Source: three-view drawing plus pictorial views. Frame: mm from the lowest corner of the part. A direction names the side the tool comes from. Give positions to 0.01 mm unless a question says otherwise; leave off trailing zeros. Order: outer loops, then holes, each group sorted by start corner. A loop starts at its lowest first (then second) coordinate and runs counter-clockwise, first axis right, second up.
1) Material intervals for line 1 (Y direction, x = 6.5, z = 12); line 2 (X direction, y = 66, z = 13); line 3 (Z direction, x = 22, y = 33), sorted ascending.
2) First-contact query: P1, Ø12, axis at x = 33, z = 15.5, coming from the -Y side. Flat tip, straight axial feed; report the tip coordinate or a pass-through.
3) Section C-C, the plane y = 22.5. Return loops of the section in (x, z).
4) Section B-B, the plane x = 30. Return loops of the section in (y, z), plus the area to 3 significant figures.
5) Draft query along X for the marked faces 4, 5 and 6. Return one class per face: released by +X, released by -X, zero draft, split by the parting line, or undercut.
6) Section A-A, the plane z = 23. Return loops of the section in (x, y), plus the area to 3 significant figures.
7) Access query for the marked faces 1, 2 and 3. Directions: +Z, -Z, +X, -X, +Y, -Y. A direction counts if a zero-diameter tool reaches every point of the face in a straight line with its end or side. Return the directions, or none.
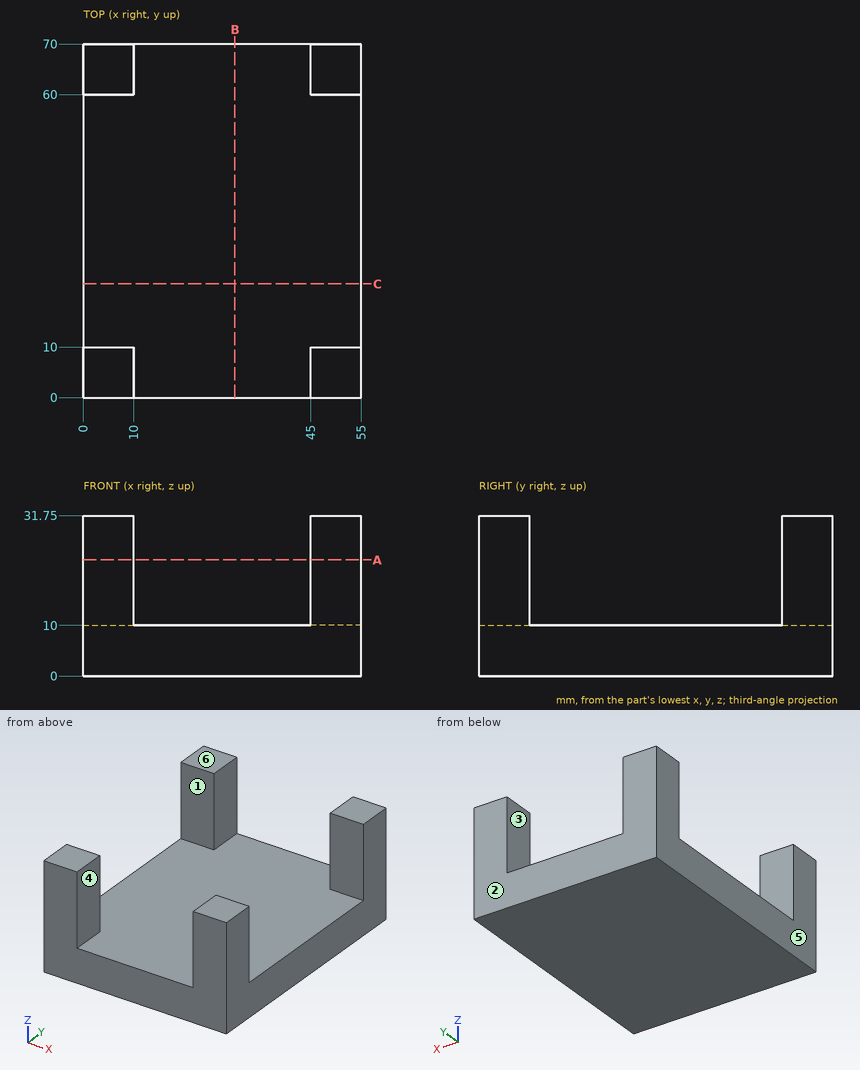
From the geometry:
1. line 1: y = 0 to 10, 60 to 70
1. line 2: x = 0 to 10, 45 to 55
1. line 3: z = 0 to 10
2. P1: stops at y = 0
3. outline: (0, 0) - (55, 0) - (55, 10) - (0, 10) - close
4. outline: (0, 0) - (70, 0) - (70, 10) - (0, 10) - close
4. area: 700 mm2
5. face 4: undercut
5. face 5: released by -X
5. face 6: zero draft
6. outline: (0, 0) - (10, 0) - (10, 10) - (0, 10) - close; (0, 60) - (10, 60) - (10, 70) - (0, 70) - close; (45, 0) - (55, 0) - (55, 10) - (45, 10) - close; (45, 60) - (55, 60) - (55, 70) - (45, 70) - close
6. area: 400 mm2
7. face 1: +Z, +X, -X
7. face 2: +Z, -Z, +X, -X, +Y
7. face 3: +Z, +Y, -Y
